Design review of the part built by this model. Coordinates are the model's own, in mm. Round coordinates to 2 decimals unless told otherwise and drop trailing zeros. Loops run counter-clockwise (first coordinate to the right, second up) from the corner with the lowest first, then second, coordinate; pieces in that order, holes last. Notation, with made-up numbers: (-39.75, 44) - (4.25, 44) arc R26 ccw to (4.25, 68) - close; hole circle Ø10 at (69.5, -2.5). An arc over 180 degrees is marked (long way). Return JSON: item names as keys, results as strings. Group by question number.
(1) Wall thickness on L1, parallel to Y at x = -71.5, z = 0.9; L2, parallel to Y at x = 57, z = 0.7; L3, parallel to Y at x = 20, z = 0.7: over which ranges is each line inside the solid? List them lowest first. Write a range as [from, to].
(2) We need section B-B, the plane x = 39.5. Write out the cut boundary in (y, z), and give its area (3 significant figures).
(3) We need section A-A, the plane x = -77.5. Write out the cut boundary in (y, z).
(4) We need section C-C, the plane z = -0.15. Give the number of separate pieces and of enclosed holes in the cut face, and give its area (3 significant figures).
(5) Clearance check with flat-ended pins moving along their axes: pin 1 (1.5 mm diameter, centred on x = 13.5, z = -1, fed in from -Y); pin 2 (1 mm diameter, centred on x = -76.5, y = -78.5, fed in from -Z); pin 3 (1 mm diameter, centred on y = 5.5, z = 0.5, fed in from -X). State where each tip first meets the part, or that it passes through.
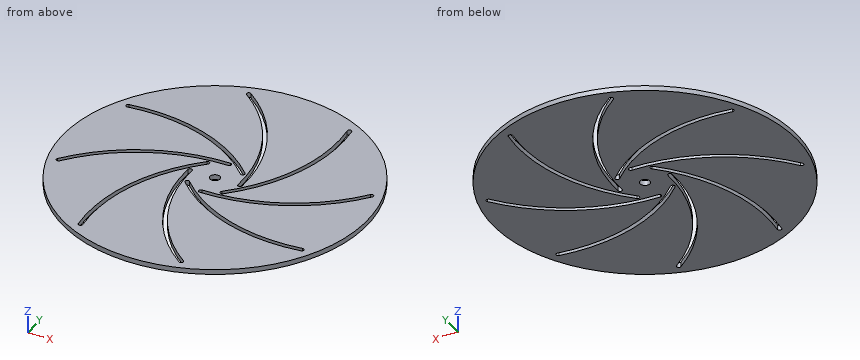
from build123d import *

# Parameters (mm, degrees)
SKETCH1_R                = 107.5
SKETCH1_R_2              = 3.5
BOSS_EXTRUDE1_DEPTH      = 1.75
BOSS_EXTRUDE1_DEPTH_BACK = 1.75


with BuildPart() as part:
    # Sketch1 → Boss-Extrude1 (new body, two sides)
    with BuildSketch(Plane.XY) as boss_extrude1_sk:
        Circle(SKETCH1_R)
        Circle(SKETCH1_R_2, mode=Mode.SUBTRACT)
        with BuildLine():
            ThreePointArc((0, 19.5), (-54.1059262, 6.549513138), (-96.484687775, -29.495))
            ThreePointArc((-96.484687775, -29.495), (-96.158582907, -31.591104867), (-94.06247804, -31.265))
            ThreePointArc((-94.06247804, -31.265), (-52.74761843, 3.874629963), (0, 16.5))
            ThreePointArc((0, 16.5), (1.5, 18), (0, 19.5))
        make_face(mode=Mode.SUBTRACT)
        with BuildLine():
            ThreePointArc((13.788582233, 13.788582233), (-33.627462165, 42.889872472), (-89.081091517, 47.368862495))
            ThreePointArc((-89.081091517, 47.368862495), (-90.33267052, 45.656101566), (-88.619909591, 44.404522563))
            ThreePointArc((-88.619909591, 44.404522563), (-34.558421561, 40.037975805), (11.66726189, 11.66726189))
            ThreePointArc((11.66726189, 11.66726189), (13.788582233, 11.66726189), (13.788582233, 13.788582233))
        make_face(mode=Mode.SUBTRACT)
        with BuildLine():
            ThreePointArc((19.5, 0), (6.549513138, 54.1059262), (-29.495, 96.484687775))
            ThreePointArc((-29.495, 96.484687775), (-31.591104867, 96.158582907), (-31.265, 94.06247804))
            ThreePointArc((-31.265, 94.06247804), (3.874629963, 52.74761843), (16.5, 0))
            ThreePointArc((16.5, 0), (18, -1.5), (19.5, 0))
        make_face(mode=Mode.SUBTRACT)
        with BuildLine():
            ThreePointArc((13.788582233, -13.788582233), (42.889872472, 33.627462165), (47.368862495, 89.081091517))
            ThreePointArc((47.368862495, 89.081091517), (45.656101566, 90.33267052), (44.404522563, 88.619909591))
            ThreePointArc((44.404522563, 88.619909591), (40.037975805, 34.558421561), (11.66726189, -11.66726189))
            ThreePointArc((11.66726189, -11.66726189), (11.66726189, -13.788582233), (13.788582233, -13.788582233))
        make_face(mode=Mode.SUBTRACT)
        with BuildLine():
            ThreePointArc((0, -19.5), (54.1059262, -6.549513138), (96.484687775, 29.495))
            ThreePointArc((96.484687775, 29.495), (96.158582907, 31.591104867), (94.06247804, 31.265))
            ThreePointArc((94.06247804, 31.265), (52.74761843, -3.874629963), (0, -16.5))
            ThreePointArc((0, -16.5), (-1.5, -18), (0, -19.5))
        make_face(mode=Mode.SUBTRACT)
        with BuildLine():
            ThreePointArc((-13.788582233, -13.788582233), (33.627462165, -42.889872472), (89.081091517, -47.368862495))
            ThreePointArc((89.081091517, -47.368862495), (90.33267052, -45.656101566), (88.619909591, -44.404522563))
            ThreePointArc((88.619909591, -44.404522563), (34.558421561, -40.037975805), (-11.66726189, -11.66726189))
            ThreePointArc((-11.66726189, -11.66726189), (-13.788582233, -11.66726189), (-13.788582233, -13.788582233))
        make_face(mode=Mode.SUBTRACT)
        with BuildLine():
            ThreePointArc((-19.5, 0), (-6.549513138, -54.1059262), (29.495, -96.484687775))
            ThreePointArc((29.495, -96.484687775), (31.591104867, -96.158582907), (31.265, -94.06247804))
            ThreePointArc((31.265, -94.06247804), (-3.874629963, -52.74761843), (-16.5, 0))
            ThreePointArc((-16.5, 0), (-18, 1.5), (-19.5, 0))
        make_face(mode=Mode.SUBTRACT)
        with BuildLine():
            ThreePointArc((-13.788582233, 13.788582233), (-42.889872472, -33.627462165), (-47.368862495, -89.081091517))
            ThreePointArc((-47.368862495, -89.081091517), (-45.656101566, -90.33267052), (-44.404522563, -88.619909591))
            ThreePointArc((-44.404522563, -88.619909591), (-40.037975805, -34.558421561), (-11.66726189, 11.66726189))
            ThreePointArc((-11.66726189, 11.66726189), (-11.66726189, 13.788582233), (-13.788582233, 13.788582233))
        make_face(mode=Mode.SUBTRACT)
    extrude(amount=BOSS_EXTRUDE1_DEPTH)
    extrude(boss_extrude1_sk.sketch, amount=-BOSS_EXTRUDE1_DEPTH_BACK)


solid = part.part
Solutions:
{
 "1": {"L1": "[-80.27, -8.02], [-4.25, 45.79], [48.79, 80.27]", "L2": "[-91.14, -48], [-44.98, -5.03], [-1.6, 91.14]", "L3": "[-105.62, -88.77], [-84.69, -37.5], [-34.17, -17.81], [-14.77, -7.08], [-2.39, 105.62]"},
 "2": {"outline": "(-99.98, -1.75) - (-44.64, -1.75) - (-44.64, 1.75) - (-99.98, 1.75) - close; (-41.53, -1.75) - (-12.78, -1.75) - (-12.78, 1.75) - (-41.53, 1.75) - close; (-9.6, -1.75) - (24.52, -1.75) - (24.52, 1.75) - (-9.6, 1.75) - close; (32.95, -1.75) - (99.98, -1.75) - (99.98, 1.75) - (32.95, 1.75) - close", "area": "648 mm^2"},
 "3": {"outline": "(-74.5, -1.75) - (-13.02, -1.75) - (-13.02, 1.75) - (-74.5, 1.75) - close; (-9.04, -1.75) - (45.59, -1.75) - (45.59, 1.75) - (-9.04, 1.75) - close; (48.6, -1.75) - (74.5, -1.75) - (74.5, 1.75) - (48.6, 1.75) - close"},
 "4": {"separate pieces": "1", "enclosed holes": "9", "area": "33,500 mm^2"},
 "5": {"pin 1": "y = -106.74", "pin 2": "through", "pin 3": "x = -107.38"}
}
